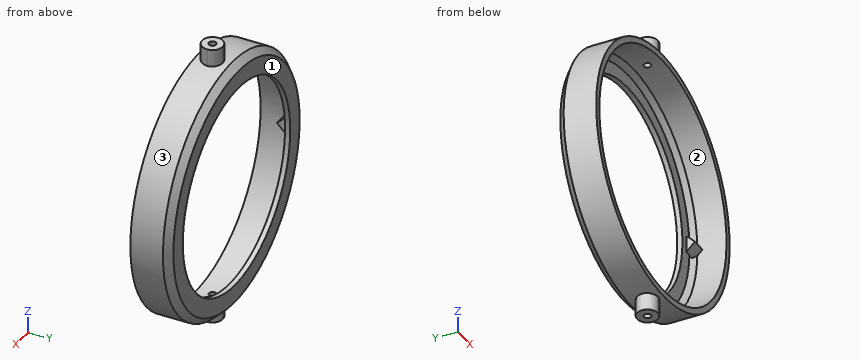
from build123d import *

# Parameters (mm, degrees)
SKETCH1_R           = 37.25
SKETCH1_R_2         = 35.5
BOSS_EXTRUDE1_DEPTH = 10
BOSS_EXTRUDE2_START = 1.5
SKETCH1_2_R         = 37.25
SKETCH1_2_R_2       = 30
BOSS_EXTRUDE2_DEPTH = 1.5
CHAMFER1_SIZE       = 1.5
CHAMFER2_SIZE       = 2
CUT_EXTRUDE1_DEPTH  = 10
BOSS_EXTRUDE4_START = 5
BOSS_EXTRUDE4_DEPTH = 6
BOSS_EXTRUDE6_START = -1
BOSS_EXTRUDE6_DEPTH = 5


with BuildPart() as part:
    # Sketch1 → Boss-Extrude1 (new body)
    with BuildSketch(Plane(origin=(0, 0, 0), x_dir=(1, 0, 0), z_dir=(0, 1, 0))):
        with Locations(Location((0, 0, 0), (0, 0, 270))):
            Circle(SKETCH1_R)
        with Locations(Location((0, 0, 0), (0, 0, 270))):
            Circle(SKETCH1_R_2, mode=Mode.SUBTRACT)
    extrude(amount=-BOSS_EXTRUDE1_DEPTH)

    # Sketch1_2 → Boss-Extrude2 (add)
    with BuildSketch(Plane(origin=(0, 0, 0), x_dir=(1, 0, 0), z_dir=(0, 1, 0)).offset(BOSS_EXTRUDE2_START)):
        with Locations(Location((0, 0, 0), (0, 0, 270))):
            Circle(SKETCH1_2_R)
        with Locations(Location((0, 0, 0), (0, 0, 270))):
            Circle(SKETCH1_2_R_2, mode=Mode.SUBTRACT)
    extrude(amount=-BOSS_EXTRUDE2_DEPTH)

    # Chamfer1
    chamfer1_edges = [part.edges().sort_by_distance(p)[0] for p in [
        (0, 0, -35.5),
    ]]
    chamfer(chamfer1_edges, length=CHAMFER1_SIZE)

    # Chamfer2
    chamfer2_edges = [part.edges().sort_by_distance(p)[0] for p in [
        (0, 1.5, -37.25),
    ]]
    chamfer(chamfer2_edges, length=CHAMFER2_SIZE)

    # Sketch2 → Cut-Extrude1 (cut)
    with BuildSketch(Plane.XY.offset(37.25)):
        with BuildLine():
            ThreePointArc((1.05, -5.5), (0.74246212, -4.75753788), (0, -4.45))
            Line((0, -4.45), (0, -6.55))
            ThreePointArc((0, -6.55), (0.74246212, -6.24246212), (1.05, -5.5))
        make_face()
        with BuildLine():
            Line((0, -6.55), (0, -4.45))
            ThreePointArc((0, -4.45), (-1.05, -5.5), (0, -6.55))
        make_face()
    cut_extrude1 = extrude(amount=-CUT_EXTRUDE1_DEPTH, mode=Mode.SUBTRACT)

    # Sketch2_3 → Boss-Extrude4 (add)
    with BuildSketch(Plane.XY.offset(37.25).offset(BOSS_EXTRUDE4_START)):
        with BuildLine():
            ThreePointArc((3.05, -5.5), (2.156675683, -3.343324317), (0, -2.45))
            Line((0, -2.45), (0, -4.45))
            ThreePointArc((0, -4.45), (0.74246212, -4.75753788), (1.05, -5.5))
            ThreePointArc((1.05, -5.5), (0.74246212, -6.24246212), (0, -6.55))
            Line((0, -6.55), (0, -8.55))
            ThreePointArc((0, -8.55), (2.156675683, -7.656675683), (3.05, -5.5))
        make_face()
        with BuildLine():
            Line((0, -4.45), (0, -2.45))
            ThreePointArc((0, -2.45), (-3.05, -5.5), (0, -8.55))
            Line((0, -8.55), (0, -6.55))
            ThreePointArc((0, -6.55), (-1.05, -5.5), (0, -4.45))
        make_face()
    boss_extrude4 = extrude(amount=-BOSS_EXTRUDE4_DEPTH)

    # Mirror1: Cut-Extrude1, Boss-Extrude4 across plane
    add(cut_extrude1.mirror(Plane.XY), mode=Mode.SUBTRACT)
    add(boss_extrude4.mirror(Plane.XY))

    # tirangle → Boss-Extrude6 (add)
    with BuildSketch(Plane(origin=(37.25, 0, 0), x_dir=(0, 0, -1), z_dir=(1, 0, 0)).offset(BOSS_EXTRUDE6_START)):
        Polygon((2.5, -0.5), (-2.5, -0.5), (0, -3), align=None)
    boss_extrude6 = extrude(amount=-BOSS_EXTRUDE6_DEPTH)

    # Mirror2: Boss-Extrude6 across plane
    add(boss_extrude6.mirror(Plane(origin=(0, 0, 0), x_dir=(0, 0, 1), z_dir=(1, 0, 0))))


solid = part.part
The model under review builds one solid part; all positions refer to its coordinate system, in mm. Face numbers are marked on the shaded views. Give positions to 0.01 mm unless a question says otherwise; leave off trailing zeros. Order: outer loops, then holes, each group sorted by start corner. A loop starts at its lowest first (then second) coordinate and runs counter-clockwise, first axis right, second up. Notation, with made-up numbers: M 13,49 L 18,49 A16 cw 18,67 Z; hole C 26.25,17.25 d2. An arc over 180 degrees is marked long. Use one line per item in the form item = value. Start each with the question number.
Item 1: Insertion check: pin 1 Ø2 at (x, y) = (8.5, -8) entering from +Z; pin 2 Ø3 at (x, z) = (28, 3) entering from +Y; pin 3 Ø6 at (y, z) = (-8.5, 7) entering from -X; pin 4 Ø3 at (y, z) = (-1.5, -0.5) entering from -X. Each pin has a flat end and moves straight along its axis. Give the tip position at first contact, or say it passes through.
Item 2: The part is to be moulded in two halves that separate along X. For the marked faces 1, 2 and 3, say which applies: pulls with the +X half, pulls with the -X half, needs draft (parallel to the pull), parting line crosses it, or undercut.
Item 3: We need section A-A on y = -7.5. Give the boundary of the cut face in (x, z).
Item 4: To check wall thickness, follow line 1 along X through (y, z) = (-7, 0); line 2 along Z through (x, y) = (0, -7); line 3 along X through (y, z) = (-4.5, 5.5). State the ranges of each line that lie inside material, in increasing order. Write a range as from..to.
Completed:
q1.pin_1 = 36.49
q1.pin_2 = through
q1.pin_3 = -37.03
q1.pin_4 = -37.25
q2.face_1 = needs draft
q2.face_2 = undercut
q2.face_3 = parting line crosses it
q3.outline = M -2.3,-42.25 L 2.3,-42.25 L 2.3,-37.18 A37.25 ccw 2.3,37.18 L 2.3,42.25 L -2.3,42.25 L -2.3,37.18 A37.25 ccw -2.3,-37.18 Z; hole C 0,0 d71
q4.line_1 = -37.25..-35.5, 35.5..37.25
q4.line_2 = -42.25..-35.5, 35.5..42.25
q4.line_3 = -36.84..-35.07, 35.07..36.84
